Source: CAD feature listing. Evaluate the final solid. Frame: model axes, mm. Coordinates: 2 decimals unless noted, no trailing zeros. Use one line per item in the form item = value. Start each with the question number.
from build123d import *

# Parameters (mm, degrees)
SKETCH1_R                = 4.7625
BOSS_EXTRUDE2_DEPTH      = 5.08
BOSS_EXTRUDE2_DEPTH_BACK = 5.08


with BuildPart() as part:
    # Sketch1 → Boss-Extrude2 (new body, two sides)
    with BuildSketch(Plane(origin=(0, 0, 0), x_dir=(1, 0, 0), z_dir=(0, 1, 0))) as boss_extrude2_sk:
        with BuildLine():
            Line((-89.802561211, 99.962561211), (89.802561211, 99.962561211))
            ThreePointArc((89.802561211, 99.962561211), (96.986766108, 96.986766108), (99.962561211, 89.802561211))
            Line((99.962561211, 89.802561211), (99.962561211, -89.802561211))
            ThreePointArc((99.962561211, -89.802561211), (96.986766108, -96.986766108), (89.802561211, -99.962561211))
            Line((89.802561211, -99.962561211), (-89.802561211, -99.962561211))
            ThreePointArc((-89.802561211, -99.962561211), (-96.986766108, -96.986766108), (-99.962561211, -89.802561211))
            Line((-99.962561211, -89.802561211), (-99.962561211, 89.802561211))
            ThreePointArc((-99.962561211, 89.802561211), (-96.986766108, 96.986766108), (-89.802561211, 99.962561211))
        make_face()
        with Locations((89.802561211, 89.802561211)):
            Circle(SKETCH1_R, mode=Mode.SUBTRACT)
        with Locations((89.802561211, -89.802561211)):
            Circle(SKETCH1_R, mode=Mode.SUBTRACT)
        with Locations((-89.802561211, -89.802561211)):
            Circle(SKETCH1_R, mode=Mode.SUBTRACT)
        with Locations((-89.802561211, 89.802561211)):
            Circle(SKETCH1_R, mode=Mode.SUBTRACT)
    extrude(amount=BOSS_EXTRUDE2_DEPTH)
    extrude(boss_extrude2_sk.sketch, amount=-BOSS_EXTRUDE2_DEPTH_BACK)


solid = part.part
(1) Material intervals for line 1 (Z direction, x = 85.5, y = -4.25), sorted ascending.
(2) Mould query, pull axis X, two halves, no side actions, for faces 1 (the face through (89.18, -0.07, 85.08)), 2 (the face through (-1, 0, -99.963)), 3 (the face through (-90.42, -0.07, 85.08)), 4 (the face through (-99.963, 0, 1)). Classes: +X half, -X half, draft (parallel to the pull), parting line (faces both ways), or undercut.
(3) Contact query for a flat-ended pin moving along its axis: pin 1 (5.5 mm diameter, centred on x = -89.8, z = -89.8, fed in from -Y). Output: stop coordinate, or through.
Recorded:
q1.line_1 = -99.96 to -91.84, -87.76 to 87.76, 91.84 to 99.96
q2.face_1 = undercut
q2.face_2 = draft
q2.face_3 = undercut
q2.face_4 = -X half
q3.pin_1 = through
